CAD build for the part. Positions are in the model's coordinates, mm. A direction names the side the tool comes from. Coordinates: 2 decimals unless noted, no trailing zeros. Loops run counter-clockwise (first coordinate to the right, second up) from the corner with the lowest first, then second, coordinate; pieces in that order, holes last.
1) Wall check: line 1 along Z through (x, y) = (28.2, -2.25); line 2 along Y through (x, z) = (22.5, 13); line 3 along Z through (x, y) = (-16, -3.5). Give the ranges that are in metal, low to high.
2) Saw through at D-D, the plane x = 28.2. Write the cut outline in (y, z), and give its area (3 significant figures).
3) Two-plate mould, pull along Y, no slides. Class faces 1 (the cylindrical face through (-21.8, -19.72, 10.93)), 2 (the flat face through (-48, -18, -17)), 3 (the cylindrical face through (10.45, -0.65, 23.98)): +Y half, -Y half, draft (parallel to the pull), parting line (faces both ways), or undercut.
4) Saw through at C-C, the plane x = -46. Write the cut outline in (y, z).
5) Saw through at A-A, the plane z = 17. Give the number of separate pieces and of enclosed holes in the cut face, and give its area (3 significant figures).
6) Pin check, flat tips, straight feed: pin 1 Ø11 at (x, y) = (-32, -14) entering from +Z; pin 2 Ø0.5 at (y, z) = (-2.5, 25) entering from -X; pin 3 Ø6.5 at (x, y) = (-23.46, -15.2) entering from -Z (3 decimals); pin 4 Ø9 at (x, y) = (-22, -14) entering from -Z. Stop position of each tip, or through.
7) Which spindle directions (+Z, -Z, +X, -X, +Y, -Y) get a long thin tool onto all of the face, cutting with end or side? Do faces 4 (the flat face through (33, -13, 22.5)), 5 (the flat face through (-21.2, -7, 0)), 6 (the flat face through (34, -13, -11.5)), 7 (the cylindrical face through (-25.91, -3.55, 16.28)). Say none if no direction does.
```python
from build123d import *

# Parameters (mm, degrees)
BOSS_EXTRUDE1_DEPTH        = 22.5
SKETCH2_W                  = 30.8
SKETCH2_H                  = 23
CUT_EXTRUDE1_DEPTH         = 65
SKETCH3_R                  = 1.6
CUT_EXTRUDE2_DEPTH         = 65
SKETCH7_R                  = 2.15
MOTOR_MOUNTING_DEPTH       = 3
SKETCH4_R                  = 4.05
BEARING_HOLE_DEPTH         = 3.625
AXLE_THRU_HOLES_DEPTH      = 71.062333854
AXLE_THRU_HOLES_DEPTH_BACK = 71.062333854
SKETCH5_R                  = 3
FILLET3_R                  = 2
TOP_MOUNT_HOLES_DEPTH      = 63.024914385
TOP_MOUNT_HOLES_DEPTH_BACK = 7
SKETCH6_R                  = 2.4
FILLET4_R                  = 3
FILLET5_START              = 22.5
FILLET5_DEPTH              = 3
FILLET5_START_2            = -13.087721306
FILLET5_2_DEPTH            = 13.087721306
FILLET5_START_3            = -22.2
FILLET5_3_DEPTH            = 9.436583025
FILLET5_4_OUTLINE_R        = 4.05
FILLET5_4_DEPTH            = 2.71686
FILLET5_5_DEPTH            = 3
FILLET5_START_4            = -22.5
FILLET5_6_DEPTH            = 45
CUT_EXTRUDE3_REACH         = 76.168
SKETCH8_R                  = 8.55


with BuildPart() as part:
    # Sketch1 → Boss-Extrude1 (new, symmetric)
    with BuildSketch(Plane.XY):
        with BuildLine():
            Line((-18.2, 0), (-34.2, 0))
            Line((-34.2, 0), (-40, -18))
            Line((-40, -18), (-52, -18))
            Line((-52, -18), (-52, -22.2))
            Line((-52, -22.2), (0, -22.2))
            Line((0, -22.2), (52, -22.2))
            Line((52, -22.2), (52, -18))
            Line((52, -18), (40, -18))
            Line((40, -18), (34.2, 0))
            Line((34.2, 0), (18.2, 0))
            ThreePointArc((18.2, 0), (0, -18.2), (-18.2, 0))
        make_face()
    extrude(amount=BOSS_EXTRUDE1_DEPTH, both=True)

    # Sketch2 → Cut-Extrude1 (cut)
    with BuildSketch(Plane(origin=(0, 0, 0), x_dir=(1, 0, 0), z_dir=(0, 1, 0))):
        with Locations((-36.6, 0)):
            Rectangle(SKETCH2_W, SKETCH2_H)
        with Locations((36.6, 0)):
            Rectangle(SKETCH2_W, SKETCH2_H)
    extrude(amount=-CUT_EXTRUDE1_DEPTH, mode=Mode.SUBTRACT)

    # Sketch3 → Cut-Extrude2 (cut)
    with BuildSketch(Plane(origin=(0, -18, 0), x_dir=(1, 0, 0), z_dir=(0, 1, 0))):
        with Locations(Location((-46, 17, 0), (0, 0, 270))):
            Circle(SKETCH3_R)
        with Locations(Location((46, 17, 0), (0, 0, 270))):
            Circle(SKETCH3_R)
        with Locations(Location((46, -17, 0), (0, 0, 180))):
            Circle(SKETCH3_R)
        with Locations(Location((-46, -17, 0), (0, 0, 180))):
            Circle(SKETCH3_R)
    extrude(amount=-CUT_EXTRUDE2_DEPTH, mode=Mode.SUBTRACT)

    # Sketch7 → Motor-Mounting (add)
    with BuildSketch(Plane.XY.offset(22.5)):
        with BuildLine():
            Line((-7.5, 0), (-8.35, 0))
            ThreePointArc((-8.35, 0), (-12.5, 4.15), (-16.65, 0))
            Line((-16.65, 0), (-18.2, 0))
            Line((-18.2, 0), (-20, 0))
            Line((-20, 0), (-20, -22.2))
            Line((-20, -22.2), (0, -22.2))
            Line((0, -22.2), (20, -22.2))
            Line((20, -22.2), (20, 0))
            Line((20, 0), (18.2, 0))
            Line((18.2, 0), (16.65, 0))
            ThreePointArc((16.65, 0), (12.5, 4.15), (8.35, 0))
            Line((8.35, 0), (7.5, 0))
            ThreePointArc((7.5, 0), (0, -7.5), (-7.5, 0))
        make_face()
        with Locations((-12.5, 0)):
            Circle(SKETCH7_R, mode=Mode.SUBTRACT)
        with Locations(Location((12.5, 0, 0), (0, 0, 180))):
            Circle(SKETCH7_R, mode=Mode.SUBTRACT)
    extrude(amount=MOTOR_MOUNTING_DEPTH)

    # Sketch4 → Bearing-Hole (cut, symmetric)
    with BuildSketch(Plane.XY.offset(22.5)):
        with Locations((-23.455543055, -15.2)):
            Circle(SKETCH4_R)
    bearing_hole = extrude(amount=BEARING_HOLE_DEPTH, both=True, mode=Mode.SUBTRACT)

    # Mirror1: Bearing-Hole across plane
    add(bearing_hole.mirror(Plane.XY), mode=Mode.SUBTRACT)

    # Sketch5 → Axle-Thru-Holes (cut, two sides: drawn at the far end of the back side and taken through both)
    with BuildSketch(Plane.XY.offset(18.875).offset(-AXLE_THRU_HOLES_DEPTH_BACK)):
        with Locations((-23.455543055, -15.2)):
            Circle(SKETCH5_R)
    extrude(amount=AXLE_THRU_HOLES_DEPTH + AXLE_THRU_HOLES_DEPTH_BACK, mode=Mode.SUBTRACT)

    # Fillet3
    fillet3_edges = [part.edges().sort_by_distance(p)[0] for p in [
        (21.2, -11.1, -11.5),
        (21.2, -11.1, 11.5),
        (-21.2, -19.689005249, 11.5),
        (-21.2, -19.689005249, -11.5),
    ]]
    fillet(fillet3_edges, radius=FILLET3_R)

    # Sketch6 → Top-Mount-Holes (cut, two sides: drawn at the far end of the back side and taken through both)
    with BuildSketch(Plane(origin=(0, 0, 0), x_dir=(1, 0, 0), z_dir=(0, 1, 0)).offset(-TOP_MOUNT_HOLES_DEPTH_BACK)):
        with Locations((-28.2, 17)):
            Circle(SKETCH6_R)
        with Locations((28.2, 17)):
            Circle(SKETCH6_R)
        with Locations(Location((28.2, -17, 0), (0, 0, 90))):
            Circle(SKETCH6_R)
        with Locations((-28.2, -17)):
            Circle(SKETCH6_R)
    extrude(amount=TOP_MOUNT_HOLES_DEPTH + TOP_MOUNT_HOLES_DEPTH_BACK, mode=Mode.SUBTRACT)

    # Fillet4
    fillet4_edges = [part.edges().sort_by_distance(p)[0] for p in [
        (40, -18, 17),
        (-40, -18, 17),
        (40, -18, -17),
        (-40, -18, -17),
    ]]
    fillet(fillet4_edges, radius=FILLET4_R)

    # Fillet5: read off the stored shape, not the designer's step
    # Fillet5 outline → Fillet5 (add)
    with BuildSketch(Plane.XY.offset(FILLET5_START)):
        with BuildLine():
            ThreePointArc((-7.5, 0), (-8.14090356, 0.498741958), (-8.530676829, 1.211186842))
            ThreePointArc((-8.530676829, 1.211186842), (-8.395417734, 0.612294391), (-8.35, 0))
            Line((-8.35, 0), (-7.5, 0))
        make_face()
        with BuildLine():
            ThreePointArc((8.530676829, 1.211186842), (8.14090356, 0.498741958), (7.5, 0))
            Line((7.5, 0), (8.35, 0))
            ThreePointArc((8.35, 0), (8.395417734, 0.612294391), (8.530676829, 1.211186842))
        make_face()
    extrude(amount=FILLET5_DEPTH)

    # Fillet5 2 outline → Fillet5 2 (add)
    with BuildSketch(Plane(origin=(0, 0, 0), x_dir=(1, 0, 0), z_dir=(0, 1, 0)).offset(FILLET5_START_2)):
        with BuildLine():
            ThreePointArc((-22, -22.5), (-20.585786438, -23.085786438), (-20, -24.5))
            Line((-20, -24.5), (-20, -22.5))
            Line((-20, -22.5), (-22, -22.5))
        make_face()
        with BuildLine():
            ThreePointArc((20, -24.5), (20.585786438, -23.085786438), (22, -22.5))
            Line((22, -22.5), (20, -22.5))
            Line((20, -22.5), (20, -24.5))
        make_face()
    extrude(amount=FILLET5_2_DEPTH)

    # Fillet5 3 outline → Fillet5 3 (add)
    with BuildSketch(Plane(origin=(0, 0, 0), x_dir=(1, 0, 0), z_dir=(0, 1, 0)).offset(FILLET5_START_3)):
        with BuildLine():
            ThreePointArc((20, -24.5), (20.585786438, -23.085786438), (22, -22.5))
            Line((22, -22.5), (20, -22.5))
            Line((20, -22.5), (20, -24.5))
        make_face()
    extrude(amount=FILLET5_3_DEPTH)

    # Fillet5 4 outline → Fillet5 4 (cut)
    with BuildSketch(Plane.XY.offset(FILLET5_START)):
        with Locations((-23.455543055, -15.2)):
            Circle(FILLET5_4_OUTLINE_R)
    extrude(amount=FILLET5_4_DEPTH, mode=Mode.SUBTRACT)

    # Fillet5 5 outline → Fillet5 5 (add)
    with BuildSketch(Plane.XY.offset(FILLET5_START)):
        with BuildLine():
            ThreePointArc((18.315711478, 0), (17.153991419, 0.371993088), (16.424423193, 1.349593496))
            ThreePointArc((16.424423193, 1.349593496), (16.593217332, 0.684157785), (16.65, 0))
            Line((16.65, 0), (18.315711478, 0))
        make_face()
        with BuildLine():
            Line((-18.315711478, 0), (-16.65, 0))
            ThreePointArc((-16.65, 0), (-16.593217332, 0.684157785), (-16.424423193, 1.349593496))
            ThreePointArc((-16.424423193, 1.349593496), (-17.153991419, 0.371993088), (-18.315711478, 0))
        make_face()
    extrude(amount=FILLET5_5_DEPTH)

    # Fillet5 6 outline → Fillet5 6 (add)
    with BuildSketch(Plane.XY.offset(FILLET5_START_4)):
        with BuildLine():
            Line((18.2, 0), (18.315711478, 0))
            ThreePointArc((18.315711478, 0), (18.257831342, 0.000837703), (18.199999692, 0.00335011))
            ThreePointArc((18.199999692, 0.00335011), (18.199999923, 0.001675055), (18.2, 0))
        make_face()
        with BuildLine():
            Line((-18.315711478, 0), (-18.2, 0))
            ThreePointArc((-18.2, 0), (-18.199999923, 0.001675055), (-18.199999692, 0.00335011))
            ThreePointArc((-18.199999692, 0.00335011), (-18.257831342, 0.000837703), (-18.315711478, 0))
        make_face()
    extrude(amount=FILLET5_6_DEPTH)

    # Cut-Extrude3: up to this face of the body (flat: up to its plane)
    cut_extrude3_end = Plane(part.part.faces().sort_by_distance((-32.525053026, -12.842804107, 22.5))[0])
    # Sketch8 → Cut-Extrude3 (cut, up to the picked face)
    with BuildSketch(Plane.XY.offset(25.5), mode=Mode.PRIVATE) as cut_extrude3_sk1:
        with Locations((-23.455543055, -15.2)):
            Circle(SKETCH8_R)
    cut_extrude3_tool1 = split(extrude(cut_extrude3_sk1.sketch, amount=-CUT_EXTRUDE3_REACH, mode=Mode.PRIVATE), bisect_by=cut_extrude3_end, keep=Keep.BOTH, mode=Mode.PRIVATE)
    add(cut_extrude3_tool1.solids().sort_by(Axis((-23.455543, -15.2, 25.5), (0, 0, -1)))[0], mode=Mode.SUBTRACT)


solid = part.part
```
Data:
1. line 1: z = -22.5 to -19.4, -14.6 to -11.5, 11.5 to 14.6, 19.4 to 22.5
1. line 2: y = -22.2 to 0
1. line 3: z = 22.5 to 25.5
2. outline: (-22.2, -22.5) - (0, -22.5) - (0, -19.4) - (-7, -19.4) - (-7, -14.6) - (0, -14.6) - (0, -11.5) - (-22.2, -11.5) - close; (-22.2, 11.5) - (0, 11.5) - (0, 14.6) - (-7, 14.6) - (-7, 19.4) - (0, 19.4) - (0, 22.5) - (-22.2, 22.5) - close
2. area: 421 mm2
3. face 1: draft
3. face 2: +Y half
3. face 3: undercut
4. outline: (-22.2, -22.5) - (-18, -22.5) - (-18, -18.6) - (-22.2, -18.6) - close; (-22.2, -15.4) - (-18, -15.4) - (-18, -11.5) - (-22.2, -11.5) - close; (-22.2, 11.5) - (-18, 11.5) - (-18, 15.4) - (-22.2, 15.4) - close; (-22.2, 18.6) - (-18, 18.6) - (-18, 22.5) - (-22.2, 22.5) - close
5. separate pieces: 3
5. enclosed holes: 1
5. area: 1,130 mm2
6. pin 1: stops at z = 22.5
6. pin 2: stops at x = -20
6. pin 3: stops at z = -18.875
6. pin 4: stops at z = -22.5
7. face 4: +Z, +X, +Y, -Y
7. face 5: -X, +Y
7. face 6: +X, +Y, -Y
7. face 7: +Y
